Autodesk Inventor part; units mm, degrees
ref_plane "YZ Plane" through (0, 0, 0) normal (1, 0, 0) x (0, 1, 0)
ref_plane "XZ Plane" through (0, 0, 0) normal (0, 1, 0) x (-1, 0, 0)
ref_plane "XY Plane" through (0, 0, 0) normal (0, 0, 1) x (1, 0, 0)
sketch "Sketch1" plane through (0, 0, 0) normal (0, 1, 0) x (-1, 0, 0)
  line L0 (0, 0) -> (-27, 0) construction
  line L1 (-27, -8) -> (0, -8)
  arc A0 (0, -8) -> (0, 8) centre (0, 0) ccw
  arc A1 (-27, 8) -> (-27, -8) centre (-27, 0) ccw
  line L2 (14.5, 10) -> (-41.5, 10)
  line L3 (-41.5, 10) -> (-41.5, -10)
  line L4 (-41.5, -10) -> (14.5, -10)
  line L5 (14.5, -10) -> (14.5, 10)
  line L6 (14.5, 10) -> (-41.5, -10) construction
  line L7 (-41.5, 10) -> (14.5, -10) construction
  line L8 (14.5, 10) -> (-41.5, 10)
  line L9 (-41.5, 10) -> (-41.5, 15)
  line L10 (-41.5, 15) -> (14.5, 15)
  line L11 (14.5, 15) -> (14.5, 10)
  arc A2 (0, -8) -> (-5.3358, 5.9607) centre (0, 0) ccw
  arc A3 (-21.6642, 5.9607) -> (-27, -8) centre (-27, 0) ccw
  line L12 (9, -10) -> (-36, -10)
  line L13 (-36, -10) -> (-36, 10) construction
  line L14 (-36, 10) -> (9, 10)
  line L15 (9, 10) -> (9, -10) construction
  line L16 (9, -10) -> (-36, 10) construction
  line L17 (-36, -10) -> (9, 10) construction
  line L18 (9, 10) -> (-6, 10)
  line L19 (-6, 10) -> (-6, 5.9607)
  line L20 (-36, 10) -> (-21, 10)
  line L21 (-21, 10) -> (-21, 5.9607)
  line L22 (-5.3358, 5.9607) -> (-21.6642, 5.9607) construction
  line L23 (-21, 5.9607) -> (-21.6642, 5.9607)
  line L24 (-6, 5.9607) -> (-5.3358, 5.9607)
  point P0 (-13.5, 0)
  point P1 (-27, 8)
  point P2 (0, 8)
  dimension "d0" = 27
  dimension "d1" = 16
  dimension "d2" = 56
  dimension "d3" = 20
  dimension "d4" = 5
  dimension "d5" = 45
  dimension "d6" = 15
  dimension "d7" = 15
extrude "Extrusion1" add sketch "Sketch1" along normal blind 8 contours L1 A0 A2 L24 L19 L2 L5 L4 L3 L21 L23 A3 A1
extrude "Extrusion2" add sketch "Sketch1" along normal blind 15.5 contours L2 L9 L10 L11
sketch "Sketch2" plane through (21, 0, 10) normal (0, 0, -1) x (-1, 0, 0)
  line L0 (35.5, 8) -> (15, 8)
  line L1 (-20.5, 8) -> (-20.5, 15.5)
  line L2 (35.5, 8) -> (-20.5, 8)
  line L3 (-20.5, 8) -> (-20.5, 15.5)
  line L4 (-20.5, 15.5) -> (35.5, 15.5)
  line L5 (35.5, 15.5) -> (35.5, 8)
  line L6 (31, 8) -> (-16, 8)
  line L7 (-16, 8) -> (-16, 12.5)
  line L8 (-16, 12.5) -> (31, 12.5)
  line L9 (31, 12.5) -> (31, 8)
  line L10 (-20.5, 8) -> (35.5, 8)
  point P0 (21, 0)
  point P1 (7.5, 8)
  dimension "d12" = 47
  dimension "d13" = 4.5
extrude "Extrusion3" add sketch "Sketch2" along normal blind 3 contours L0 L9 L8 L7 L2 L1 L4 L5
sketch "Sketch3" plane through (41.5, 0, -10) normal (0, 0, -1) x (-1, 0, 0)
  circle A0 centre (52, 4) radius 2.15
  line L0 (56, 0) -> (56, 8)
  line L1 (0, 0) -> (56, 0)
  circle A1 centre (4, 4) radius 2.15
  line L2 (0, 0) -> (0, 8)
  point P0 (41.5, 0)
  dimension "d16" = 4.3
  dimension "d17" = 4
  dimension "d18" = 4
  dimension "d19" = 4.3
  dimension "d20" = 4
  dimension "d21" = 4
extrude "Extrusion4" cut sketch "Sketch3" against normal blind 32
sketch "Sketch5" plane through (0, 8, 0) normal (0, 1, 0) x (1, 0, 0)
  line L0 (-14.5, 10) -> (-14.5, -15)
  line L1 (41.5, 10) -> (-14.5, 10)
  line L2 (-14.5, 0) -> (41.5, 0)
  line L3 (41.5, 0) -> (41.5, 10)
  line L4 (41.5, 10) -> (-14.5, 10)
  line L5 (-14.5, 10) -> (-14.5, 0)
  point P0 (0, 0)
extrude "Extrusion6" cut sketch "Sketch5" against normal blind 10
properties part number "Ultrasonic_sensor_frame_Buttom"
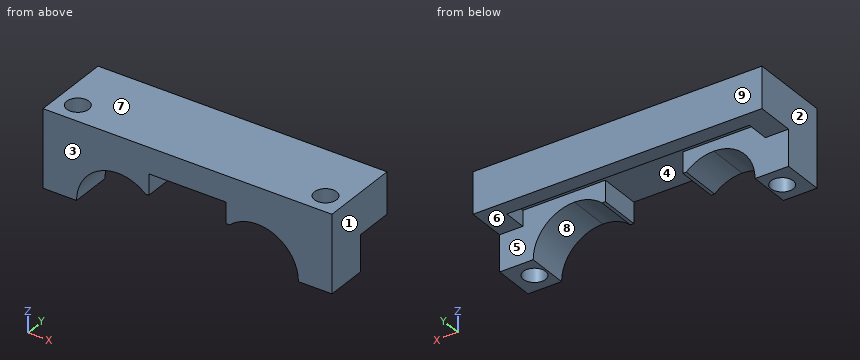
Verification items for the finished model (mm, model axes). Face numbers are marked on the shaded views. A direction names the side the tool comes from. Coordinates: 2 decimals unless noted, no trailing zeros. Loops run counter-clockwise (first coordinate to the right, second up) from the corner with the lowest first, then second, coordinate; pieces in that order, holes last. Notation, with made-up numbers: (-34, -36) -> (15, -36) arc R29 ccw to (15, -12) -> close; hole circle Ø6 at (-35, -3.75). An arc over 180 degrees is marked (long way). Answer in a Markdown table with one row per item. Add a question column.
1. Section check D-D, the plane z = 13.25. Enter the section's corners in (x, y).
2. Draft check along X on the marked faces 1, 2, 3 and 4. Enter one of: +X half, -X half, draft (parallel to the pull), parting line (faces both ways), or undercut.
3. Material ranges on probe 1 along Y at (x, z) = (-10.5, 7.25); probe 2 along Y at (x, z) = (35, 9.25); probe 3 along X at (y, z) = (12, 9.25), recorded low to high. Write a range as [from, to].
4. Section check A-A, the plane x = 37.5. Enter the section's corners in (y, z), then the cut area to 4 significant figures.
5. Depth check by flat-ended pin: P1, Ø6, axis at x = 15, y = 5.5, coming from the -Z side; P2, Ø0.7, axis at x = 21, y = 3.5, coming from the -Z side; P3, Ø5, axis at x = 32.5, z = 2.5, coming from the +Y side; P4, Ø4, axis at x = -10.5, y = 4, coming from the +Z side. Enter the tip coordinate at first touch or a pass-through.
6. Section check C-C, the plane y = 9.25. Enter the section's corners in (x, z), then the cut area to 3 significant figures.
7. Access from +Z, -Z, +X, -X, +Y, -Y to the whole of each face (thin tool, end or side, straight path). Record for the marked faces 5, 6, 7, 8 and 9.
8. Section check B-B, the plane z = 4. Enter the section's corners in (x, y), then the cut area to 3 significant figures.
Derived:
| question | item | result |
|---|---|---|
| 1 | outline | (-14.5, 0) -> (41.5, 0) -> (41.5, 15.5) -> (-14.5, 15.5) -> close; hole circle Ø4.3 at (-10.5, 4); hole circle Ø4.3 at (37.5, 4) |
| 2 | face 1 | +X half |
| 2 | face 2 | -X half |
| 2 | face 3 | draft |
| 2 | face 4 | undercut |
| 3 | probe 1 | y = [0, 1.85], [6.15, 15.5] |
| 3 | probe 2 | y = [0, 8], [12.5, 15.5] |
| 3 | probe 3 | x = [-14.5, -10], [37, 41.5] |
| 4 | outline | (0, 0) -> (1.85, 0) -> (1.85, 15) -> (0, 15) -> close; (6.15, 0) -> (8, 0) -> (8, 7) -> (15.5, 7) -> (15.5, 15) -> (6.15, 15) -> close |
| 4 | area | 115.5 mm² |
| 5 | P1 | stops at z = 10 |
| 5 | P2 | stops at z = 5.96 |
| 5 | P3 | stops at y = 8 |
| 5 | P4 | passes through |
| 6 | outline | (-14.5, 7) -> (-10, 7) -> (-10, 10) -> (37, 10) -> (37, 7) -> (41.5, 7) -> (41.5, 15) -> (-14.5, 15) -> close |
| 6 | area | 307 mm² |
| 7 | face 5 | -Z |
| 7 | face 6 | -Z, +X, -X, +Y |
| 7 | face 7 | +Z, +X, -X, +Y, -Y |
| 7 | face 8 | -Z, -Y |
| 7 | face 9 | +Z, -Z, +X, -X, +Y |
| 8 | outline | (-14.5, 0) -> (-6.93, 0) -> (-6.93, 8) -> (-14.5, 8) -> close; (33.93, 0) -> (41.5, 0) -> (41.5, 8) -> (33.93, 8) -> close; hole circle Ø4.3 at (-10.5, 4); hole circle Ø4.3 at (37.5, 4) |
| 8 | area | 92.1 mm² |
